Geometry check sheet. Reference: the model listing, model coordinates, mm. Face numbers are marked on the shaded views. A direction names the side the tool comes from. Coordinates: 2 decimals unless noted, no trailing zeros. Loops run counter-clockwise (first coordinate to the right, second up) from the corner with the lowest first, then second, coordinate; pieces in that order, holes last. Notation, with made-up numbers: (85.25, -4.75) - (95.25, -4.75) arc R32 ccw to (95.25, 23.25) - close; hole circle Ø8 at (7.25, -20.5). An arc over 180 degrees is marked (long way). One line per item, written item: value.
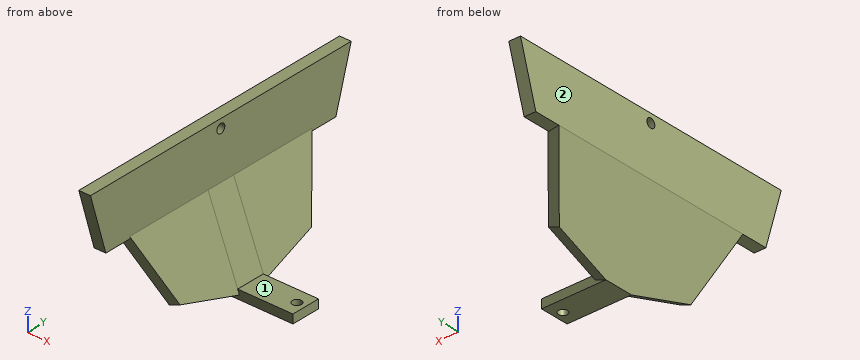
from build123d import *

# Parameters (mm, degrees)
EXTRUDE_1_DEPTH     = 10
SKETCH_2_R          = 1.55
CUT_EXTRUDE_3_DEPTH = 10
SKETCH_3_R          = 1.55
CUT_EXTRUDE_4_DEPTH = 10
EXTRUDE_2_DEPTH     = 4
EXTRUDE_START       = -4
EXTRUDE_4_OUTLINE_R = 1.55
EXTRUDE_4_DEPTH     = 4


# Read off the part's stored shape, not the designer's step: the extrude step
with BuildPart() as part:
    # Sketch 1 → Extrude 1 (new body)
    with BuildSketch(Plane(origin=(0, 0, 0), x_dir=(1, 0, 0), z_dir=(0, 1, 0))):
        Polygon((0, 0), (3, 0), (3, 16.697011668), (14.11903113, 45), (33, 45), (33, 48), (11, 48), (0, 20), align=None)
    extrude(amount=EXTRUDE_1_DEPTH)

    # Sketch 2 → Cut-Extrude 3 (cut)
    with BuildSketch(Plane.ZY):
        with Locations((-3, 5)):
            Circle(SKETCH_2_R)
    extrude(amount=-CUT_EXTRUDE_3_DEPTH, mode=Mode.SUBTRACT)

    # Sketch 3 → Cut-Extrude 4 (cut)
    with BuildSketch(Plane(origin=(0, 0, -48), x_dir=(-1, 0, 0), z_dir=(0, 0, -1))):
        with Locations((-30, 5)):
            Circle(SKETCH_3_R)
    extrude(amount=-CUT_EXTRUDE_4_DEPTH, mode=Mode.SUBTRACT)

    # Sketch 4 → Extrude 2 (add)
    with BuildSketch(Plane(origin=(-6.806629834, 0, -2.674033149), x_dir=(-0.36565237242299337, 0, 0.9307514934403471), z_dir=(-0.9307514934403471, 0, -0.36565237242299337))):
        Polygon((-18.615029869, 10), (-18.615029869, 41), (-42.698247782, 30.73), (-48.698247782, 10), (-48.698247782, 0), (-42.698247782, -20.73), (-18.615029869, -31), align=None)
    extrude(amount=-EXTRUDE_2_DEPTH)

    # Extrude 4 outline → Extrude 4 (add)
    with BuildSketch(Plane.ZY.offset(EXTRUDE_START)):
        Polygon((-20, -40), (0, -46), (0, 56), (-20, 50), align=None)
        with Locations((-3, 5)):
            Circle(EXTRUDE_4_OUTLINE_R, mode=Mode.SUBTRACT)
    extrude(amount=EXTRUDE_4_DEPTH)


solid = part.part
(1) Access from +Z, -Z, +X, -X, +Y, -Y to the whole of each face (thin tool, end or side, straight path). Record for the marked faces 1 and 2.
Reply:
face 1: +Z, +X, +Y, -Y
face 2: +Z, -Z, -X, +Y, -Y
(2) Cross-section at D-D on x = 21. Record the cut outline in (y, z).
Reply:
outline: (0, -48) - (10, -48) - (10, -45) - (0, -45) - close
(3) Cross-section at A-A on y = 5. Record the cut outline in (x, z).
Reply:
outline: (0, -20) - (11, -48) - (28.45, -48) - (28.45, -45) - (14.12, -45) - (4, -19.24) - (4, -4.55) - (0, -4.55) - close; (0, -1.45) - (4, -1.45) - (4, 0) - (0, 0) - close; (31.55, -48) - (33, -48) - (33, -45) - (31.55, -45) - close
(4) Cross-section at B-B on x = 30. Record the cut outline in (y, z).
Reply:
outline: (0, -48) - (3.45, -48) - (3.45, -45) - (0, -45) - close; (6.55, -48) - (10, -48) - (10, -45) - (6.55, -45) - close
(5) Material ranges on probe 1 along Y at (x, z) = (30, -45.65); probe 2 along X at (y, z) = (-14.5, -17); probe 3 along X at (y, z) = (33, -23.5) (3 decimals), recorded low to high. Write a range as from..to.
Reply:
probe 1: 0..3.45, 6.55..10
probe 2: 0..4
probe 3: 1.375..5.673
(6) Cross-section at C-C on z = -3. Record the cut outline in (x, y).
Reply:
outline: (0, -45.1) - (4, -45.1) - (4, 3.45) - (0, 3.45) - close; (0, 6.55) - (4, 6.55) - (4, 55.1) - (0, 55.1) - close
(7) Go/stop test with flat-tipped pins: pin 1 Ø3 at (x, y) = (1.5, 47) entering from -Z; pin 2 Ø3 at (y, z) = (-21, -39) entering from +X; pin 3 Ø3.5 at (x, z) = (18, -47) entering from +Y; pin 4 Ø3 at (x, y) = (16.5, -13) entering from -Z. Record where each tip stops, or that it passes through.
Reply:
pin 1: z = -20
pin 2: x = 12.35
pin 3: y = 10
pin 4: through
